```python
from build123d import *

# Parameters (mm, degrees)
SKETCH1_W           = 8.9916
SKETCH1_H           = 14.5034
BOSS_EXTRUDE1_DEPTH = 10.9982
SKETCH2_R           = 3.357740144
CUT_EXTRUDE1_DEPTH  = 11.43
SKETCH3_W           = 8.9916
SKETCH3_H           = 10.9982
CUT_EXTRUDE2_DEPTH  = 0.254
FILLET1_R           = 2.54
FILLET2_R           = 2.54


with BuildPart() as part:
    # Sketch1 → Boss-Extrude1 (new body)
    with BuildSketch(Plane(origin=(0, 0, 0), x_dir=(1, 0, 0), z_dir=(0, 1, 0))):
        with Locations((4.4958, 7.2517)):
            Rectangle(SKETCH1_W, SKETCH1_H)
    extrude(amount=BOSS_EXTRUDE1_DEPTH)

    # Sketch2 → Cut-Extrude1 (cut)
    with BuildSketch(Plane.XY):
        with Locations((4.4958, 6.5024)):
            Circle(SKETCH2_R)
    extrude(amount=-CUT_EXTRUDE1_DEPTH, mode=Mode.SUBTRACT)

    # Sketch3 → Cut-Extrude2 (cut)
    with BuildSketch(Plane(origin=(0, 10.9982, 0), x_dir=(1, 0, 0), z_dir=(0, 1, 0))):
        with Locations((4.4958, 9.0043)):
            Rectangle(SKETCH3_W, SKETCH3_H)
    extrude(amount=-CUT_EXTRUDE2_DEPTH, mode=Mode.SUBTRACT)

    # Fillet1
    fillet1_edges = [part.edges().sort_by_distance(p)[0] for p in [
        (8.9916, 10.7442, -9.0043),
    ]]
    fillet(fillet1_edges, radius=FILLET1_R)

    # Fillet2
    fillet2_edges = [part.edges().sort_by_distance(p)[0] for p in [
        (0, 10.7442, -9.0043),
    ]]
    fillet(fillet2_edges, radius=FILLET2_R)


solid = part.part
```
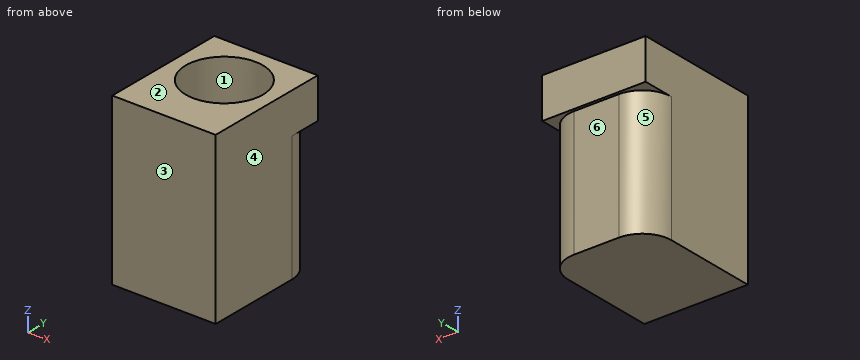
The model under review builds one solid part; all positions refer to its coordinate system, in mm. Face numbers are marked on the shaded views. A direction names the side the tool comes from. Round coordinates to 2 decimals unless told otherwise and drop trailing zeros. Loops run counter-clockwise (first coordinate to the right, second up) from the corner with the lowest first, then second, coordinate; pieces in that order, holes last. Notation, with made-up numbers: M -29,-7 L -3,-7 A12 ccw -3,9 Z; hole C 15,58 d5. An arc over 180 degrees is marked long. Put each result on its own line as item: value.
Q1. Consider section D-D, the plane x = 5.25. Give the boundary of the cut face in (y, z), then the cut area to 3 significant figures.
Result set:
outline: M 0,-14.5 L 10.74,-14.5 L 10.74,-3.51 L 11,-3.51 L 11,0 L 9.77,0 L 9.77,-11.43 L 3.23,-11.43 L 3.23,0 L 0,0 Z
area: 81.9 mm²
Q2. Consider section A-A, the plane z = -1. Give the boundary of the cut face in (x, y), then the cut area to 3 significant figures.
Result set:
outline: M 0,0 L 8.99,0 L 8.99,11 L 0,11 Z; hole C 4.5,6.5 d6.72
area: 63.5 mm²
Q3. Mouldability with a two-part tool opening along Y and no side actions: class the marked faces 1, 2 and 3 as released by +Y, released by -Y, zero draft, split by the parting line, or undercut.
Result set:
face 1: undercut
face 2: zero draft
face 3: released by -Y
Q4. To check wall thickness, follow L1, parallel to Y at x = 4, z = -13.25; L2, parallel to Z at x = 3.75, y = 5.25; L3, parallel to Y at x = 3.5, z = -7.5. State the ranges of each line that lie inside material, in increasing order.
Result set:
L1: y = 0 to 10.74
L2: z = -14.5 to -11.43
L3: y = 0 to 3.3, 9.71 to 10.74
Q5. Consider section C-C, the plane x = 7.25. Give the boundary of the cut face in (y, z), then the cut area to 3 significant figures.
Result set:
outline: M 0,-14.5 L 10.62,-14.5 L 10.62,-3.51 L 11,-3.51 L 11,0 L 8.42,0 L 8.42,-11.43 L 4.58,-11.43 L 4.58,0 L 0,0 Z
area: 111 mm²
Q6. Consider section B-B, the plane y = 5. Give the boundary of the cut face in (x, z), then the cut area to 3 significant figures.
Result set:
outline: M 0,-14.5 L 8.99,-14.5 L 8.99,0 L 7.5,0 L 7.5,-11.43 L 1.49,-11.43 L 1.49,0 L 0,0 Z
area: 61.8 mm²
Q7. For pin 1 (1.2 mm diameter, centred on x = 4.5, z = -9.5, fed in from +Y), flat-tipped, find the tip position at first contact; note if it passes through.
Result set:
pin 1: stops at y = 10.74
Q8. Machinability: for the marked faces 4, 5 and 6, which of the approach directions +Z, -Z, +X, -X, +Y, -Y give a long, thin tool a straight path to every point of the face, cutting with its end or side? Answer none if there is none.
Result set:
face 4: +Z, -Z, +X, +Y, -Y
face 5: -Z, -X, +Y
face 6: -Z, +X, -X, +Y
